Work out the finished part from the listing and answer in its coordinate system (mm). Round coordinates to 2 decimals unless told otherwise and drop trailing zeros. Order: outer loops, then holes, each group sorted by start corner. A loop starts at its lowest first (then second) coordinate and runs counter-clockwise, first axis right, second up. Notation, with made-up numbers: M -28.5,39 L -19.5,39 A22 cw -19.5,63 Z; hole C -6,41 d6. An arc over 180 degrees is marked long. Return JSON: item names as keys, results as strings.
from build123d import *

# Parameters (mm, degrees)
SKETCH1_W           = 1518.68
SKETCH1_H           = 829.31
BOSS_EXTRUDE1_DEPTH = 6.35
CUT_EXTRUDE1_REACH  = 1732.371
SKETCH2_W           = 870
SKETCH2_H           = 230
SKETCH2_W_2         = 1240.954831331
SKETCH2_H_2         = 207.299090818
SKETCH2_W_3         = 335.086201595
SKETCH2_H_3         = 262.200219892


with BuildPart() as part:
    # Sketch1 → Boss-Extrude1 (new body)
    with BuildSketch(Plane(origin=(0, 0, 0), x_dir=(1, 0, 0), z_dir=(0, 1, 0))):
        with Locations((759.34, 414.655)):
            Rectangle(SKETCH1_W, SKETCH1_H)
    extrude(amount=BOSS_EXTRUDE1_DEPTH)

    # Sketch2 → Cut-Extrude1 (cut, up to next)
    with BuildSketch(Plane(origin=(0, 6.35, 0), x_dir=(1, 0, 0), z_dir=(0, 1, 0)), mode=Mode.PRIVATE) as cut_extrude1_sk1:
        with Locations((525, 205)):
            Rectangle(SKETCH2_W, SKETCH2_H)
    cut_extrude1_tool1 = extrude(cut_extrude1_sk1.sketch, amount=-CUT_EXTRUDE1_REACH, mode=Mode.PRIVATE) & part.part
    # Sketch2 → Cut-Extrude1 (cut, up to next)
    with BuildSketch(Plane(origin=(0, 6.35, 0), x_dir=(1, 0, 0), z_dir=(0, 1, 0)), mode=Mode.PRIVATE) as cut_extrude1_sk2:
        with Locations((660.423310547, 665.496365601)):
            Rectangle(SKETCH2_W_2, SKETCH2_H_2)
    cut_extrude1_tool2 = extrude(cut_extrude1_sk2.sketch, amount=-CUT_EXTRUDE1_REACH, mode=Mode.PRIVATE) & part.part
    # Sketch2 → Cut-Extrude1 (cut, up to next)
    with BuildSketch(Plane(origin=(0, 6.35, 0), x_dir=(1, 0, 0), z_dir=(0, 1, 0)), mode=Mode.PRIVATE) as cut_extrude1_sk3:
        with Locations((1279.95415502, 213.035336328)):
            Rectangle(SKETCH2_W_3, SKETCH2_H_3)
    cut_extrude1_tool3 = extrude(cut_extrude1_sk3.sketch, amount=-CUT_EXTRUDE1_REACH, mode=Mode.PRIVATE) & part.part
    add(cut_extrude1_tool1.solids().sort_by_distance((525, 6.35, -205))[0], mode=Mode.SUBTRACT)
    add(cut_extrude1_tool2.solids().sort_by_distance((660.423311, 6.35, -665.496366))[0], mode=Mode.SUBTRACT)
    add(cut_extrude1_tool3.solids().sort_by_distance((1279.954155, 6.35, -213.035336))[0], mode=Mode.SUBTRACT)


solid = part.part
Item 1: Find section D-D (x = 638). Determine the outline of the cut face in (y, z), plus the area to 3 significant figures.
Output:
{"outline": "M 0,-829.31 L 6.35,-829.31 L 6.35,-769.15 L 0,-769.15 Z; M 0,-561.85 L 6.35,-561.85 L 6.35,-320 L 0,-320 Z; M 0,-90 L 6.35,-90 L 6.35,0 L 0,0 Z", "area": "2,490 mm^2"}
Item 2: Find section B-B (y = 4.5). Determine the outline of the cut face in (x, z), plus the area to 3 significant figures.
Output:
{"outline": "M 0,-829.31 L 1518.68,-829.31 L 1518.68,0 L 0,0 Z; hole M 39.95,-769.15 L 1280.9,-769.15 L 1280.9,-561.85 L 39.95,-561.85 Z; hole M 90,-320 L 960,-320 L 960,-90 L 90,-90 Z; hole M 1112.41,-344.14 L 1447.5,-344.14 L 1447.5,-81.94 L 1112.41,-81.94 Z", "area": "714,000 mm^2"}
Item 3: Find section C-C (z = -685.5). Determine the outline of the cut face in (x, y).
Output:
{"outline": "M 0,0 L 39.95,0 L 39.95,6.35 L 0,6.35 Z; M 1280.9,0 L 1518.68,0 L 1518.68,6.35 L 1280.9,6.35 Z"}
Item 4: Find section A-A (x = 1398). Determine the outline of the cut face in (y, z), plus the area to 3 significant figures.
Output:
{"outline": "M 0,-829.31 L 6.35,-829.31 L 6.35,-344.14 L 0,-344.14 Z; M 0,-81.94 L 6.35,-81.94 L 6.35,0 L 0,0 Z", "area": "3,600 mm^2"}
Item 5: Consider line 1 along Z through (x, y) = (1262, 3.25); line 2 along Z through (x, y) = (294, 3.75); line 3 along X through (y, z) = (4.75, -204). Determine where each line is inside the solid, lowest interval first. Write a range as [from, to].
Output:
{"line 1": "z = [-829.31, -769.15], [-561.85, -344.14], [-81.94, 0]", "line 2": "z = [-829.31, -769.15], [-561.85, -320], [-90, 0]", "line 3": "x = [0, 90], [960, 1112.41], [1447.5, 1518.68]"}
